from build123d import *

# Parameters (mm, degrees)
F0_R          = 0.5
F1_DEPTH      = 10
F0_R_2        = 0.75
F2_DEPTH      = 0.25
F3_R          = 0.1
F5_DEPTH      = 25
F5_DEPTH_BACK = 25
F7_DEPTH      = 25
F7_DEPTH_BACK = 25


with BuildPart() as f1:
    # F0 (on Top) → F1 (new body)
    with BuildSketch(Plane.XY):
        Circle(F0_R)
    extrude(amount=F1_DEPTH)

    # F0 (on Top) → F2 (join)
    with BuildSketch(Plane.XY):
        Circle(F0_R_2)
        Circle(F0_R, mode=Mode.SUBTRACT)
        Circle(F0_R)
    extrude(amount=-F2_DEPTH)

    # F3
    f3_edges = [f1.edges().sort_by_distance(p)[0] for p in [
        (-0.75, 0, -0.25),
    ]]
    fillet(f3_edges, radius=F3_R)

    # F4 (on Right) → F5 (cut, two sides)
    with BuildSketch(Plane.YZ) as f5_sk:
        Polygon((-0.677386, 8.761818), (0, 10.000281), (0.69153, 8.720125), (0.69153, 10.707485), (-0.809413, 10.707485), align=None)
    extrude(amount=F5_DEPTH, mode=Mode.SUBTRACT)
    extrude(f5_sk.sketch, amount=-F5_DEPTH_BACK, mode=Mode.SUBTRACT)

    # F6 (on Front) → F7 (cut, two sides)
    with BuildSketch(Plane.XZ) as f7_sk:
        Polygon((-0.791911, 8.716712), (0, 10.009787), (0.678298, 8.74771), (0.678298, 10.293201), (-0.791911, 10.293201), align=None)
    extrude(amount=F7_DEPTH, mode=Mode.SUBTRACT)
    extrude(f7_sk.sketch, amount=-F7_DEPTH_BACK, mode=Mode.SUBTRACT)


solid = f1.part
Source: CAD feature listing. Evaluate the final solid. Frame: model axes, mm. A direction names the side the tool comes from. Coordinates: 2 decimals unless noted, no trailing zeros. Loops run counter-clockwise (first coordinate to the right, second up) from the corner with the lowest first, then second, coordinate; pieces in that order, holes last. Notation, with made-up numbers: (51, 19.5) - (97, 19.5) arc R25 ccw to (97, 48.5) - close; hole circle Ø6 at (59, 74). An arc over 180 degrees is marked (long way). Return JSON: item names as keys, results as strings.
Q1. Access query for faces 1 (the flat face through (0, 0, -0.25)), 2 (the cylindrical face through (-0.108, -0.488, 4.633)). Directions: +Z, -Z, +X, -X, +Y, -Y. A direction counts if a zero-diameter tool reaches every point of the face in a straight line with its end or side. Return the directions, or none.
Results:
{"face 1": "-Z, +X, -X, +Y, -Y", "face 2": "+Z"}
Q2. Section A-A, the plane z = 2.75. Return loops of the section in (x, y), plus the area to 3 significant figures.
Results:
{"outline": "circle Ø1 at (0, 0)", "area": "0.785 mm2"}
Q3. Material intervals for line 1 along Z through (x, y) = (0.5, 0.4); line 2 along X through (y, z) = (0.05, 0.75), sorted ascending.
Results:
{"line 1": "-0.25 to 0", "line 2": "-0.5 to 0.5"}
